Verification items for this drawing (mm, ordinates from the low corner). A direction names the side the tool comes from. Round coordinates to 2 decimals unless told otherwise and drop trailing zeros. Order: outer loops, then holes, each group sorted by start corner. A loop starts at its lowest first (then second) coordinate and runs counter-clockwise, first axis right, second up. Notation, with made-up numbers: (16.5, 72) -> (70.5, 72) arc R19 ccw to (70.5, 93) -> close; hole circle Ø4 at (58, 19.5). An arc over 180 degrees is marked (long way). Put each result on its own line as item: value.
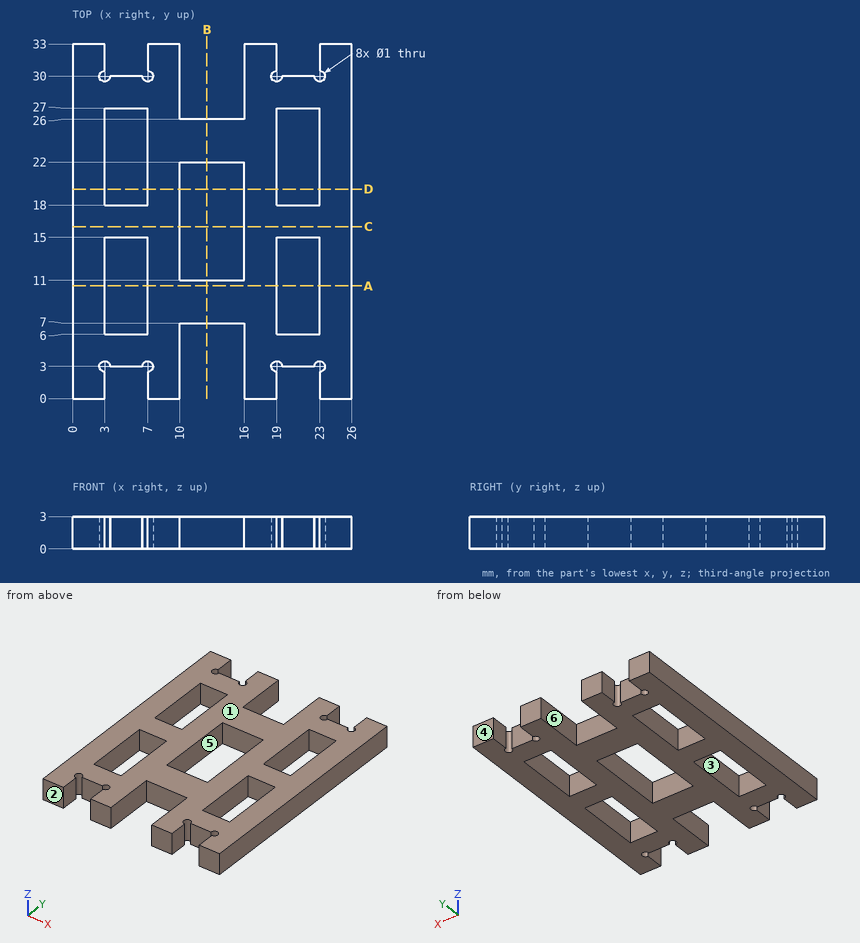
Item 1: Section check D-D on y = 19.5. Record the boundary of the cut face in (x, z), then the cut area to 3 significant figures.
Check sheet entries:
outline: (0, 0) -> (3, 0) -> (3, 3) -> (0, 3) -> close; (7, 0) -> (10, 0) -> (10, 3) -> (7, 3) -> close; (16, 0) -> (19, 0) -> (19, 3) -> (16, 3) -> close; (23, 0) -> (26, 0) -> (26, 3) -> (23, 3) -> close
area: 36.0 mm^2
Item 2: Section check C-C on y = 16. Record the boundary of the cut face in (x, z).
Check sheet entries:
outline: (0, 0) -> (10, 0) -> (10, 3) -> (0, 3) -> close; (16, 0) -> (26, 0) -> (26, 3) -> (16, 3) -> close
Item 3: Gauge pin test, flat ends, axial feed: pin 1 Ø1.5 at (x, z) = (21, 1.5) entering from -Y; pin 2 Ø1.5 at (x, z) = (20.5, 2) entering from +Y; pin 3 Ø0.9 at (x, y) = (3, 3) entering from +Z. Record the tip position at first contact, or that the pin passes through.
Check sheet entries:
pin 1: stops at y = 3
pin 2: stops at y = 30
pin 3: passes through
Item 4: Section check A-A on y = 10.5. Record the boundary of the cut face in (x, z).
Check sheet entries:
outline: (0, 0) -> (3, 0) -> (3, 3) -> (0, 3) -> close; (7, 0) -> (19, 0) -> (19, 3) -> (7, 3) -> close; (23, 0) -> (26, 0) -> (26, 3) -> (23, 3) -> close
Item 5: Section check B-B on x = 12.5. Record the boundary of the cut face in (y, z), then the cut area to 3 significant figures.
Check sheet entries:
outline: (7, 0) -> (11, 0) -> (11, 3) -> (7, 3) -> close; (22, 0) -> (26, 0) -> (26, 3) -> (22, 3) -> close
area: 24.0 mm^2
Item 6: Release check for a two-part mould opening along Y. For the marked faces 1, 2 and 3 record: +Y half, -Y half, draft (parallel to the pull), parting line (faces both ways), or undercut.
Check sheet entries:
face 1: draft
face 2: -Y half
face 3: undercut
Item 7: Material ranges on L1, parallel to X at y = 2, z = 0.25; L2, parallel to Y at x = 21.25, z = 0.45; L3, parallel to X at y = 9.5, z = 0.45, recorded low to high. Write a range as [from, to].
Check sheet entries:
L1: x = [0, 3], [7, 10], [16, 19], [23, 26]
L2: y = [3, 6], [15, 18], [27, 30]
L3: x = [0, 3], [7, 19], [23, 26]
Item 8: Tool access check on the marked faces 4, 5 and 6. Record the directions out of +Z, -Z, +X, -X, +Y, -Y that give a thin tool (end or side, any length) a straight path to the whole face; none if there is none.
Check sheet entries:
face 4: +Z, -Z, +X, -X, +Y
face 5: +Z, -Z
face 6: +Z, -Z, +Y
